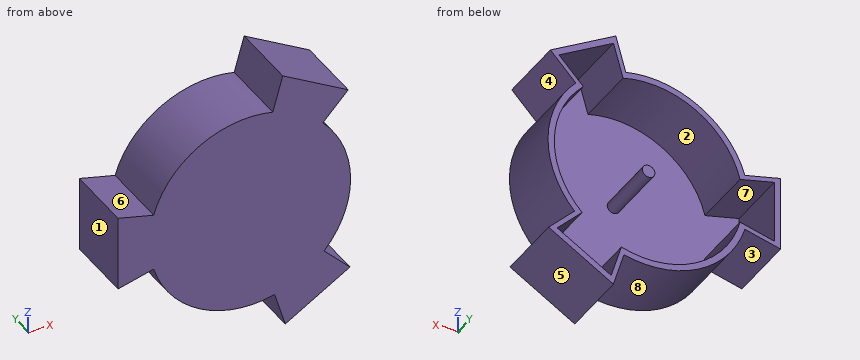
from build123d import *

# Parameters (mm, degrees)
EXTRUDE_1_DEPTH = 25.4
EXTRUDE_START   = -2.54
EXTRUDE_3_DEPTH = 2.54
SKETCH_3_R      = 2.54
EXTRUDE_4_DEPTH = 25.4


with BuildPart() as part:
    # Sketch 2 → Extrude 1 (new body)
    with BuildSketch(Plane(origin=(0, 0, 0), x_dir=(1, 0, 0), z_dir=(0, 1, 0))):
        with BuildLine():
            Line((-38.937567428, 11.639391857), (-53.34, 15.24))
            Line((-53.34, 15.24), (-53.34, -15.24))
            Line((-53.34, -15.24), (-38.937567428, -11.639391857))
            ThreePointArc((-38.937567428, -11.639391857), (-20.39841157, -35.149884857), (9.2123832, -39.582086804))
            Line((9.2123832, -39.582086804), (13.231701545, -53.873326185))
            Line((13.231701545, -53.873326185), (39.695843447, -38.751170473))
            Line((39.695843447, -38.751170473), (29.424096964, -28.032697299))
            ThreePointArc((29.424096964, -28.032697299), (40.638229061, -0.379392686), (29.942341184, 27.478460736))
            Line((29.942341184, 27.478460736), (40.412412109, 38.003291273))
            Line((40.412412109, 38.003291273), (14.235214892, 53.616898987))
            Line((14.235214892, 53.616898987), (9.949778446, 39.403191608))
            ThreePointArc((9.949778446, 39.403191608), (-20.069382693, 35.338781506), (-38.937567428, 11.639391857))
        make_face()
        with BuildLine():
            Line((10.998151919, 36.478084576), (15.115514017, 50.134331909))
            Line((15.115514017, 50.134331909), (36.929845031, 37.122992148))
            Line((36.929845031, 37.122992148), (26.870409141, 27.010944311))
            ThreePointArc((26.870409141, 27.010944311), (35.180765969, 14.626130926), (38.1, 0))
            ThreePointArc((38.1, 0), (35.042691409, -14.953921854), (26.361428934, -27.507909127))
            Line((26.361428934, -27.507909127), (36.230318646, -37.806004957))
            Line((36.230318646, -37.806004957), (14.176867061, -50.407801384))
            Line((14.176867061, -50.407801384), (10.315185941, -36.677062846))
            ThreePointArc((10.315185941, -36.677062846), (-19.123510847, -32.953017053), (-36.962429256, -9.240607314))
            Line((-36.962429256, -9.240607314), (-50.8, -12.7))
            Line((-50.8, -12.7), (-50.8, 12.7))
            Line((-50.8, 12.7), (-36.962429256, 9.240607314))
            ThreePointArc((-36.962429256, 9.240607314), (-18.815046274, 33.130107662), (10.998151919, 36.478084576))
        make_face(mode=Mode.SUBTRACT)
    extrude(amount=EXTRUDE_1_DEPTH)

    # Sketch 2_4 → Extrude 3 (add)
    with BuildSketch(Plane(origin=(0, 0, 0), x_dir=(1, 0, 0), z_dir=(0, 1, 0)).offset(EXTRUDE_START)):
        with BuildLine():
            Line((-38.937567428, 11.639391857), (-53.34, 15.24))
            Line((-53.34, 15.24), (-53.34, -15.24))
            Line((-53.34, -15.24), (-38.937567428, -11.639391857))
            ThreePointArc((-38.937567428, -11.639391857), (-20.39841157, -35.149884857), (9.2123832, -39.582086804))
            Line((9.2123832, -39.582086804), (13.231701545, -53.873326185))
            Line((13.231701545, -53.873326185), (39.695843447, -38.751170473))
            Line((39.695843447, -38.751170473), (29.424096964, -28.032697299))
            ThreePointArc((29.424096964, -28.032697299), (40.638229061, -0.379392686), (29.942341184, 27.478460736))
            Line((29.942341184, 27.478460736), (40.412412109, 38.003291273))
            Line((40.412412109, 38.003291273), (14.235214892, 53.616898987))
            Line((14.235214892, 53.616898987), (9.949778446, 39.403191608))
            ThreePointArc((9.949778446, 39.403191608), (-20.069382693, 35.338781506), (-38.937567428, 11.639391857))
        make_face()
    extrude(amount=EXTRUDE_3_DEPTH)

    # Sketch 3 → Extrude 4 (add)
    with BuildSketch(Plane(origin=(0, 0, 0), x_dir=(1, 0, 0), z_dir=(0, 1, 0))):
        with Locations(Location((0, 0, 0), (0, 0, 270))):
            Circle(SKETCH_3_R)
    extrude(amount=EXTRUDE_4_DEPTH)


solid = part.part
Geometry check sheet. Reference: the model listing, model coordinates, mm. Face numbers are marked on the shaded views. A direction names the side the tool comes from. Round coordinates to 2 decimals unless told otherwise and drop trailing zeros. Loops run counter-clockwise (first coordinate to the right, second up) from the corner with the lowest first, then second, coordinate; pieces in that order, holes last.
Item 1: Cross-section at D-D on z = 23. Record the boundary of the cut face in (x, y).
Item 2: Gauge pin test, flat ends, axial feed: pin 1 (3 mm diameter, centred on y = 12.5, z = -24, fed in from -X); pin 2 (1.5 mm diameter, centred on x = -36, y = 9.5, fed in from -Z); pin 3 (5 mm diameter, centred on y = 3, z = 34.5, fed in from -X). Record the tip position at first contact, or that the pin passes through.
Item 3: Mould release check, pull along Z, two halves, no side actions. Record for the marked faces 1, 2 and 3: pulls with the +Z half, pulls with the -Z half, needs draft (parallel to the pull), parting line crosses it, or undercut.
Item 4: Thickness scan on line 1 (Z direction, x = 33, y = 12); line 2 (Y direction, x = -6, z = 19); line 3 (Z direction, x = 28, y = 9). Record the ranges inside material, lowest first.
Item 5: Cross-section at B-B on x = 0. Record the boundary of the cut face in (y, z), then the cut area to 3 significant figures.
Item 6: Access from +Z, -Z, +X, -X, +Y, -Y to the whole of each face (thin tool, end or side, straight path). Record for the marked faces 4, 5, 6, 7 and 8.
Item 7: Cross-section at C-C on z = 44.5. Record the boundary of the cut face in (x, y), then the cut area to 3 significant figures.
Item 8: Cross-section at A-A on y = 14. Record the boundary of the cut face in (x, z).
Answer sheet:
1. outline: (-33.51, -2.54) - (33.51, -2.54) - (33.51, 25.4) - (30.37, 25.4) - (30.37, 0) - (-30.37, 0) - (-30.37, 25.4) - (-33.51, 25.4) - close
2. pin 1: stops at x = -33.84
2. pin 2: stops at z = -20.22
2. pin 3: stops at x = -25.05
3. face 1: needs draft
3. face 2: undercut
3. face 3: pulls with the -Z half
4. line 1: z = -42.42 to -39.47, -33.17 to -30.55, -23.72 to -19.04, 19.04 to 23.72, 31.76 to 34.44, 39.65 to 42.58
4. line 2: y = -2.54 to 0
4. line 3: z = -45.41 to -42.45, -28.15 to -25.84, 25.84 to 29.22, 42.51 to 45.43
5. outline: (-2.54, -40.64) - (25.4, -40.64) - (25.4, -38.1) - (0, -38.1) - (0, -2.54) - (25.4, -2.54) - (25.4, 2.54) - (0, 2.54) - (0, 38.1) - (25.4, 38.1) - (25.4, 40.64) - (-2.54, 40.64) - close
5. area: 465 mm2
6. face 4: +X, +Y, -Y
6. face 5: -Z, +X, +Y, -Y
6. face 6: +Z, +Y, -Y
6. face 7: +Y
6. face 8: -Z, +Y, -Y
7. outline: (10.6, -2.54) - (29.64, -2.54) - (29.64, 25.4) - (24.52, 25.4) - (24.52, 0) - (12.52, 0) - (12.52, 25.4) - (10.6, 25.4) - close
7. area: 227 mm2
8. outline: (-53.34, -15.24) - (-38.94, -11.64) arc R40.64 ccw to (9.95, -39.4) - (14.24, -53.62) - (40.41, -38) - (29.94, -27.48) arc R40.64 ccw to (29.42, 28.03) - (39.7, 38.75) - (13.23, 53.87) - (9.21, 39.58) arc R40.64 ccw to (-38.94, 11.64) - (-53.34, 15.24) - close; circle Ø5.08 at (0, 0); hole (-50.8, -12.7) - (-36.96, -9.24) arc R38.1 ccw to (11, -36.48) - (15.12, -50.13) - (36.93, -37.12) - (26.87, -27.01) arc R38.1 ccw to (26.36, 27.51) - (36.23, 37.81) - (14.18, 50.41) - (10.32, 36.68) arc R38.1 ccw to (-36.96, 9.24) - (-50.8, 12.7) - close
